```python
from build123d import *

# Parameters (mm, degrees)
SKETCH1_R      = 12.7
EXTRUDE1_DEPTH = 63.5
EXTRUDE2_START = -14
EXTRUDE2_DEPTH = 28


with BuildPart() as part:
    # Sketch1 → Extrude1 (new, symmetric)
    with BuildSketch(Plane.XY):
        Circle(SKETCH1_R)
    extrude(amount=EXTRUDE1_DEPTH, both=True)

    # Sketch4 → 3/8-16 Tapped Hole1 (revolve, cut)
    with BuildSketch(Plane(origin=(0, 0, 63.5), x_dir=(0, -1, 0), z_dir=(1, 0, 0))):
        Polygon((0, 0), (0, 27.784665582), (3.96875, 25.4), (3.96875, 1.42875), (5.3975, 0), align=None)
    f_3_8_16_tapped_hole1 = revolve(axis=Axis((0, 0, 69.85), (0, 0, -1)), mode=Mode.SUBTRACT)

    # Mirror1: 3/8-16 Tapped Hole1 across plane
    add(f_3_8_16_tapped_hole1.mirror(Plane.XY), mode=Mode.SUBTRACT)

    # Extrude2: read off the stored shape, not the designer's step
    # Extrude2 outline → Extrude2 (cut)
    with BuildSketch(Plane(origin=(0, 0, 0), x_dir=(1, 0, 0), z_dir=(0, 1, 0)).offset(EXTRUDE2_START)):
        with BuildLine():
            ThreePointArc((12.700884003, -62.02241801), (0.000451762, -63.309499998), (-12.699998846, -62.022599265))
            Line((-12.699998846, -62.022599265), (-14, -61.756405759))
            Line((-14, -61.756405759), (-14, -63.5))
            Line((-14, -63.5), (14, -63.5))
            Line((14, -63.5), (14, -61.756386435))
            Line((14, -61.756386435), (12.700884003, -62.02241801))
        make_face()
        with BuildLine():
            Line((-14, 63.5), (-14, 61.756405693))
            Line((-14, 61.756405693), (-12.700001857, 62.022598648))
            ThreePointArc((-12.700001857, 62.022598648), (0.000449638, 63.309499998), (12.700882852, 62.022418245))
            Line((12.700882852, 62.022418245), (14, 61.756386459))
            Line((14, 61.756386459), (14, 63.5))
            Line((14, 63.5), (-14, 63.5))
        make_face()
    extrude(amount=EXTRUDE2_DEPTH, mode=Mode.SUBTRACT)


solid = part.part
```
CAD build for the part. Positions are in the model's coordinates, mm. A direction names the side the tool comes from. Coordinates: 2 decimals unless noted, no trailing zeros. Order: outer loops, then holes, each group sorted by start corner. A loop starts at its lowest first (then second) coordinate and runs counter-clockwise, first axis right, second up. Notation, with made-up numbers: (19, 5) - (31, 5) arc R11 ccw to (31, 24) - close; hole circle Ø4 at (-34.75, 81.25). An arc over 180 degrees is marked (long way). Answer in a Markdown table with one row per item.
1. Drill centre lines: L1, parallel to X at y = 0, z = 50.25; L2, parallel to Z at x = 0.5, y = -6.5. Where is each one in solid material? Low to high. Write a range as from..to.
Answer:
| item | result |
|---|---|
| L1 | -12.7..-3.97, 3.97..12.7 |
| L2 | -63.31..63.31 |
2. Pull direction Y, two halves, no side cores. Call faces 3 (the face through (3.874, 0.86, 50.253)), 4 (the face through (-2.75, -12.4, 0.9)): +Y half, -Y half, draft (parallel to the pull), parting line (faces both ways), or undercut.
Answer:
| item | result |
|---|---|
| face 3 | undercut |
| face 4 | parting line |
3. Flat gauge pins, fed straight in: P1, Ø3, axis at x = 7, z = 44, coming from the +Y side; P2, Ø1, axis at x = 7, z = 23, coming from the -Y side; P3, Ø3, axis at x = -7, y = -3.5, coming from the -Z side. Where does each tip first touch, or does it go through?
Answer:
| item | result |
|---|---|
| P1 | y = 11.45 |
| P2 | y = -10.91 |
| P3 | z = -63.07 |
4. Slice it at B-B, the plane x = -6.5. List the corners of the cut face in (y, z).
Answer:
| item | result |
|---|---|
| outline | (-10.91, -62.97) - (10.91, -62.97) - (10.91, 62.97) - (-10.91, 62.97) - close |
5. Slice it at A-A, the plane z = -32.5. List the corners of the cut face in (x, y), then the cut area to 3 significant figures.
Answer:
| item | result |
|---|---|
| outline | circle Ø25.4 at (0, 0) |
| area | 507 mm² |
6. Slice it at C-C, the plane y = 10.5. List the corners of the cut face in (x, z), then the cut area to 3 significant figures.
Answer:
| item | result |
|---|---|
| outline | (-7.14, -62.91) arc R63.31 ccw to (7.14, -62.91) - (7.14, 62.91) arc R63.31 ccw to (-7.14, 62.91) - close |
| area | 1,810 mm² |
7. 3-axis set-ups, long thin cutter, end or side, ignore diameter. For faces 1 (the face through (-5.5, -0.22, 63.07)), 2 (the face through (3.874, 0.86, -50.253)): which of +Z, -Z, +X, -X, +Y, -Y reach the whole face in a straight line?
Answer:
| item | result |
|---|---|
| face 1 | +Z, +Y, -Y |
| face 2 | -Z |
